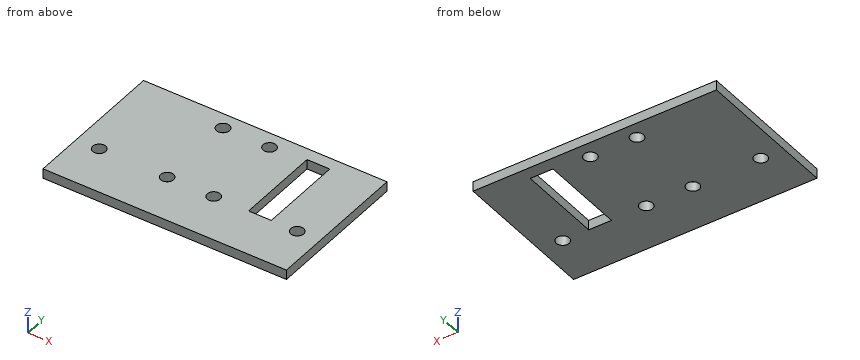
from build123d import *

# Parameters (mm, degrees)
SKETCH1_W           = 75
SKETCH1_H           = 40
SKETCH1_R           = 2
SKETCH1_W_2         = 7
SKETCH1_H_2         = 26.182038529
BOSS_EXTRUDE1_DEPTH = 3
SKETCH2_W           = 75
SKETCH2_H           = 5
BOSS_EXTRUDE2_DEPTH = 3


with BuildPart() as part:
    # Sketch1 → Boss-Extrude1 (new body)
    with BuildSketch(Plane.XY):
        Rectangle(SKETCH1_W, SKETCH1_H)
        with Locations((-30.5, -10)):
            Circle(SKETCH1_R, mode=Mode.SUBTRACT)
        with Locations((30.5, -10)):
            Circle(SKETCH1_R, mode=Mode.SUBTRACT)
        with Locations((4.771003885, 15)):
            Circle(SKETCH1_R, mode=Mode.SUBTRACT)
        with Locations((4.771003885, -10)):
            Circle(SKETCH1_R, mode=Mode.SUBTRACT)
        with Locations((-9.583817368, -10)):
            Circle(SKETCH1_R, mode=Mode.SUBTRACT)
        with Locations((-9.583817368, 15)):
            Circle(SKETCH1_R, mode=Mode.SUBTRACT)
        with Locations((19, 3.091019264)):
            Rectangle(SKETCH1_W_2, SKETCH1_H_2, mode=Mode.SUBTRACT)
    extrude(amount=BOSS_EXTRUDE1_DEPTH)

    # Sketch2 → Boss-Extrude2 (add)
    with BuildSketch(Plane.XY):
        with Locations((0, -22.5)):
            Rectangle(SKETCH2_W, SKETCH2_H)
    extrude(amount=BOSS_EXTRUDE2_DEPTH)


solid = part.part
Geometry check sheet. Reference: the model listing, model coordinates, mm. Coordinates: 2 decimals unless noted, no trailing zeros. Write each loop counter-clockwise with the first axis right and the second up, starting at its lowest first coordinate (ties: lowest second). Pieces come first, ordered by that corner, then holes. Notation, with made-up numbers: (-23, 85) -> (-14, 85) arc R14 ccw to (-14, 105) -> close; hole circle Ø9 at (89, 22). An arc over 180 degrees is marked (long way). One line per question, with ' | ' between items.
1. Cross-section at B-B on y = 15. Record the cut outline in (x, z).
Answers:
outline: (-37.5, 0) -> (-11.58, 0) -> (-11.58, 3) -> (-37.5, 3) -> close; (-7.58, 0) -> (2.77, 0) -> (2.77, 3) -> (-7.58, 3) -> close; (6.77, 0) -> (15.5, 0) -> (15.5, 3) -> (6.77, 3) -> close; (22.5, 0) -> (37.5, 0) -> (37.5, 3) -> (22.5, 3) -> close
2. Depth check by flat-ended pin: pin 1 Ø6.5 at (x, y) = (4.77, 15) entering from -Z. Enter the tip coordinate at first touch or a pass-through.
Answers:
pin 1: stops at z = 0
3. Cross-section at D-D on x = 30.5. Record the cut outline in (y, z).
Answers:
outline: (-25, 0) -> (-12, 0) -> (-12, 3) -> (-25, 3) -> close; (-8, 0) -> (20, 0) -> (20, 3) -> (-8, 3) -> close
4. Cross-section at C-C on x = 17.5. Record the cut outline in (y, z), and give its area (3 significant figures).
Answers:
outline: (-25, 0) -> (-10, 0) -> (-10, 3) -> (-25, 3) -> close; (16.18, 0) -> (20, 0) -> (20, 3) -> (16.18, 3) -> close | area: 56.5 mm²
5. Cross-section at A-A on z = 0.85. Record the cut outline in (x, y), and give its area (3 significant figures).
Answers:
outline: (-37.5, -25) -> (37.5, -25) -> (37.5, 20) -> (-37.5, 20) -> close; hole circle Ø4 at (-30.5, -10); hole circle Ø4 at (-9.58, -10); hole circle Ø4 at (-9.58, 15); hole circle Ø4 at (4.77, -10); hole circle Ø4 at (4.77, 15); hole (15.5, -10) -> (22.5, -10) -> (22.5, 16.18) -> (15.5, 16.18) -> close; hole circle Ø4 at (30.5, -10) | area: 3,120 mm²
6. Thickness scan on probe 1 along Y at (x, z) = (-30.5, 2.45); probe 2 along X at (y, z) = (3, 0.3); probe 3 along Y at (x, z) = (-9, 1.45). Record the ranges inside material, lowest first. Write a range as from..to.
Answers:
probe 1: y = -25..-12, -8..20 | probe 2: x = -37.5..15.5, 22.5..37.5 | probe 3: y = -25..-11.91, -8.09..13.09, 16.91..20
